Design review of the part built by this model. Coordinates are the model's own, in mm. Face numbers are marked on the shaded views. Round coordinates to 2 decimals unless told otherwise and drop trailing zeros. Write each loop counter-clockwise with the first axis right and the second up, starting at its lowest first coordinate (ties: lowest second). Pieces come first, ordered by that corner, then holes. Notation, with made-up numbers: (-27, -15) - (25, -15) arc R24 cw to (25, 18) - close; hole circle Ø7 at (87.5, 10.5). An arc over 180 degrees is marked (long way). Use one line per item in the form item = value.
```python
from build123d import *

# Parameters (mm, degrees)
F0_R     = 13.0048
F1_DEPTH = 20.0025
F2_DEPTH = 5.9944
F0_R_2   = 5.9944
F3_DEPTH = 13.0048


with BuildPart() as f1:
    # F0 (on Front) → F1 (new body, symmetric)
    with BuildSketch(Plane.XZ):
        with BuildLine():
            ThreePointArc((-12.949346, -21.392276), (12.278025, -21.784516), (25.0063, 0))
            ThreePointArc((25.0063, 0), (13.394448, 21.116434), (-10.657017, 22.621738))
            ThreePointArc((-10.657017, 22.621738), (-24.972454, 1.300611), (-12.949346, -21.392276))
        make_face()
        Circle(F0_R, mode=Mode.SUBTRACT)
    extrude(amount=F1_DEPTH, both=True)

    # F0 (on Front) → F2 (join, symmetric)
    with BuildSketch(Plane.XZ):
        with BuildLine():
            ThreePointArc((-12.949346, -21.392276), (-24.972454, 1.300611), (-10.657017, 22.621738))
            Line((-10.657017, 22.621738), (-99.305738, -19.140344))
            ThreePointArc((-99.305738, -19.140344), (-87.7625, -19.862798), (-82.189519, -29.9974))
            ThreePointArc((-82.189519, -29.9974), (-94.191019, -41.9989), (-106.192519, -29.9974))
            Line((-106.192519, -29.9974), (-106.192519, -70.0024))
            ThreePointArc((-106.192519, -70.0024), (-94.191019, -58.0009), (-82.189519, -70.0024))
            ThreePointArc((-82.189519, -70.0024), (-83.15941, -74.728879), (-85.912321, -78.691425))
            Line((-85.912321, -78.691425), (-27.427604, -22.968569))
            ThreePointArc((-27.427604, -22.968569), (-20.455258, -19.730028), (-12.949346, -21.392276))
        make_face()
    extrude(amount=F2_DEPTH, both=True)

    # F0 (on Front) → F3 (join, symmetric)
    with BuildSketch(Plane.XZ):
        with BuildLine():
            ThreePointArc((-82.189519, -29.9974), (-87.7625, -19.862798), (-99.305738, -19.140344))
            ThreePointArc((-99.305738, -19.140344), (-104.325621, -23.568881), (-106.192519, -29.9974))
            ThreePointArc((-106.192519, -29.9974), (-94.191019, -41.9989), (-82.189519, -29.9974))
        make_face()
        with Locations((-94.191019, -29.9974)):
            Circle(F0_R_2, mode=Mode.SUBTRACT)
        with BuildLine():
            ThreePointArc((-106.192519, -70.0024), (-98.917498, -81.034009), (-85.912321, -78.691425))
            ThreePointArc((-85.912321, -78.691425), (-83.15941, -74.728879), (-82.189519, -70.0024))
            ThreePointArc((-82.189519, -70.0024), (-94.191019, -58.0009), (-106.192519, -70.0024))
        make_face()
        with Locations((-94.191019, -70.0024)):
            Circle(F0_R_2, mode=Mode.SUBTRACT)
    extrude(amount=F3_DEPTH, both=True)


solid = f1.part
```
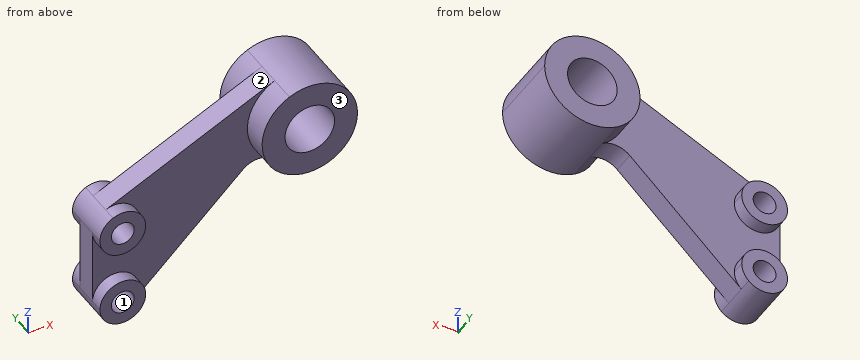
Q1. Draft analysis for pull direction X (two halves, no side actions). For the marked faces 1, 2 and 3, state which applies: released by +X, released by -X, zero draft, split by the parting line, or undercut.
Calculated:
face_1 = undercut
face_2 = released by -X
face_3 = zero draft
Q2. For P1, Ø12, axis at y = -10.5, z = -63.5, coming from the +X side; P2, Ø12, axis at x = -7, y = 12.5, coming from the -Z side; P3, Ø12, axis at x = -89.5, z = -72, coming from the -Y side, all flat-tipped, find the tip position at first contact; note any pin that passes through.
Calculated:
P1 = -65.81
P2 = -24.99
P3 = -13
Q3. We need section C-C on z = -10. Write out the cut boundary in (x, y), then the cut area to 3 significant figures.
Calculated:
outline = (-79.9, -5.99) - (-22.92, -5.99) - (-22.92, -20) - (-8.31, -20) - (-8.31, 20) - (-22.92, 20) - (-22.92, 5.99) - (-79.9, 5.99) - close; (8.31, -20) - (22.92, -20) - (22.92, 20) - (8.31, 20) - close
area = 1,850 mm2
Q4. To check wall thickness, follow line 1 along Z through (x, y) = (-95, 2.5); line 2 along Z through (x, y) = (0, 7.5); line 3 along Y through (x, z) = (-38.5, -33). State the ranges of each line that lie inside material, in increasing order. Write a range as from..to.
Calculated:
line_1 = -81.98..-75.94, -64.06..-35.94, -24.06..-17.11
line_2 = -25.01..-13, 13..25.01
line_3 = -5.99..5.99
Q5. We need section D-D on z = 17.5. Write out the cut boundary in (x, y), then the cut area to 3 significant figures.
Calculated:
outline = (-21.53, -5.99) - (-17.86, -5.99) - (-17.86, -20) - (17.86, -20) - (17.86, 20) - (-17.86, 20) - (-17.86, 5.99) - (-21.53, 5.99) - close
area = 1,470 mm2
Q6. We need section B-B on x = 0. Write out the cut boundary in (y, z), then the cut area to 3 significant figures.
Calculated:
outline = (-20, -25.01) - (20, -25.01) - (20, -13) - (-20, -13) - close; (-20, 13) - (20, 13) - (20, 25.01) - (-20, 25.01) - close
area = 960 mm2
Q7. We need section A-A on y = 8. Write out the cut boundary in (x, z), then the cut area to 3 significant figures.
Calculated:
outline = circle Ø24 at (-94.19, -30); (-85.91, -78.69) arc R12 ccw to (-82.19, -70) arc R12 ccw (long way) to start; circle Ø50.01 at (0, 0); hole circle Ø11.99 at (-94.19, -70); hole circle Ø11.99 at (-94.19, -30); hole circle Ø26.01 at (0, 0)
area = 2,110 mm2
